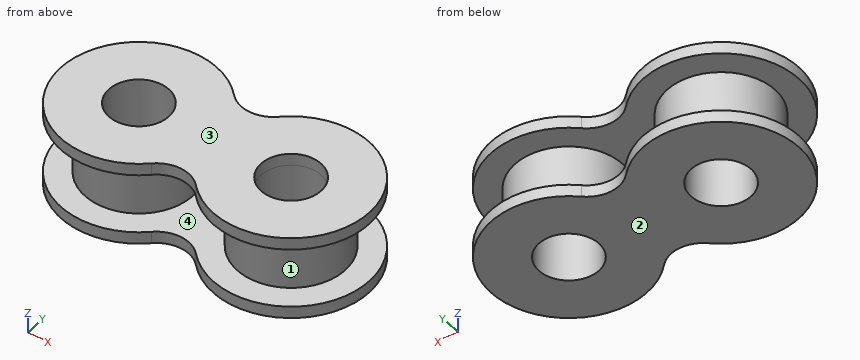
from build123d import *

# Parameters (mm, degrees)
CROQUIS1_R              = 2.5
SALIENTE_EXTRUIR1_DEPTH = 1
CROQUIS2_R              = 4.5
CROQUIS2_R_2            = 2.5
SALIENTE_EXTRUIR2_DEPTH = 5


with BuildPart() as part:
    # Croquis1 → Saliente-Extruir1 (new body)
    with BuildSketch(Plane.XY):
        with BuildLine():
            ThreePointArc((-1.903805922, 4.596194078), (-13, 0), (-1.903805922, -4.596194078))
            ThreePointArc((-1.903805922, -4.596194078), (0, -3.807611845), (1.903805922, -4.596194078))
            ThreePointArc((1.903805922, -4.596194078), (13, 0), (1.903805922, 4.596194078))
            ThreePointArc((1.903805922, 4.596194078), (0, 3.807611845), (-1.903805922, 4.596194078))
        make_face()
        with Locations((-6.5, 0)):
            Circle(CROQUIS1_R, mode=Mode.SUBTRACT)
        with Locations((6.5, 0)):
            Circle(CROQUIS1_R, mode=Mode.SUBTRACT)
    saliente_extruir1 = extrude(amount=SALIENTE_EXTRUIR1_DEPTH)

    # Croquis2 → Saliente-Extruir2 (add)
    with BuildSketch(Plane.XY.offset(1)):
        with Locations((6.5, 0)):
            Circle(CROQUIS2_R)
        with Locations((6.5, 0)):
            Circle(CROQUIS2_R_2, mode=Mode.SUBTRACT)
        with Locations((-6.5, 0)):
            Circle(CROQUIS2_R)
        with Locations((-6.5, 0)):
            Circle(CROQUIS2_R_2, mode=Mode.SUBTRACT)
    extrude(amount=SALIENTE_EXTRUIR2_DEPTH)

    # Simetría1: Saliente-Extruir1 across plane
    add(saliente_extruir1.mirror(Plane.XY.offset(3.5)))


solid = part.part
Can you work these out from the model? Positions are in its coordinate system, mm. Face numbers are marked on the shaded views. A direction names the side the tool comes from. Round coordinates to 2 decimals unless told otherwise and drop trailing zeros. Write each loop counter-clockwise with the first axis right and the second up, starting at its lowest first coordinate (ties: lowest second). Pieces come first, ordered by that corner, then holes. Notation, with made-up numbers: (6, 11.25) -> (19, 11.25) arc R7 cw to (19, 18.25) -> close; hole circle Ø1 at (-11, 45). An arc over 180 degrees is marked (long way). Use one line per item in the form item = value. Start each with the question number.
Q1. Which directions (+Z, -Z, +X, -X, +Y, -Y) give clear straight access to the entire face, cutting with the end or side of a thin tool? Please do the marked faces 3 and 4.
Q2. Imagine slicing it at C-C (z = 6.75). Please give me the cut outline in (x, y), then the cut area to 3 significant figures.
Q3. Imagine slicing it at D-D (y = 3.25). Please give me the cut outline in (x, z), then the cut area to 3 significant figures.
Q4. We'd pull the mould along X, two halves only. Please class the marked faces 1 and 2: +X half, -X half, draft (parallel to the pull), parting line (faces both ways), or undercut.
Q5. Imagine slicing it at B-B (x = 6.5). Please give me the cut outline in (y, z), then the cut area to 3 significant figures.
Q6. Imagine slicing it at A-A (y = -0.75). Please give me the cut outline in (x, z).
Q7. I'm going to push flat-ended pins straight in: P1, Ø2, axis at x = 9.5, z = 6, coming from the +Y side; P2, Ø4, axis at x = 6.5, y = 0, coming from the +Z side. Where does each tip first touch, or does it pass through?
Q8. If I drill on probe 1 along Z at (x, y) = (-2, 4.5); probe 2 along X at (y, z) = (-2, 5); probe 3 along Y at (x, z) = (6.5, 3.8), over which ranges is the centre line in solid material (lowest first)? Write a range as [from, to].
Worked out:
q1.face_3 = +Z, +X, -X, +Y, -Y
q1.face_4 = none
q2.outline = (-1.9, -4.6) arc R2.69 cw to (1.9, -4.6) arc R6.5 ccw (long way) to (1.9, 4.6) arc R2.69 cw to (-1.9, 4.6) arc R6.5 ccw (long way) to start; hole circle Ø5 at (-6.5, 0); hole circle Ø5 at (6.5, 0)
q2.area = 233 mm^2
q3.outline = (-12.13, 0) -> (12.13, 0) -> (12.13, 1) -> (9.61, 1) -> (9.61, 6) -> (12.13, 6) -> (12.13, 7) -> (-12.13, 7) -> (-12.13, 6) -> (-9.61, 6) -> (-9.61, 1) -> (-12.13, 1) -> close; hole (-3.39, 1) -> (3.39, 1) -> (3.39, 6) -> (-3.39, 6) -> close
q3.area = 111 mm^2
q4.face_1 = undercut
q4.face_2 = draft
q5.outline = (-6.5, 0) -> (-2.5, 0) -> (-2.5, 7) -> (-6.5, 7) -> (-6.5, 6) -> (-4.5, 6) -> (-4.5, 1) -> (-6.5, 1) -> close; (2.5, 0) -> (6.5, 0) -> (6.5, 1) -> (4.5, 1) -> (4.5, 6) -> (6.5, 6) -> (6.5, 7) -> (2.5, 7) -> close
q5.area = 36.0 mm^2
q6.outline = (-12.96, 0) -> (-8.88, 0) -> (-8.88, 7) -> (-12.96, 7) -> (-12.96, 6) -> (-10.94, 6) -> (-10.94, 1) -> (-12.96, 1) -> close; (-4.12, 0) -> (4.12, 0) -> (4.12, 7) -> (-4.12, 7) -> close; (8.88, 0) -> (12.96, 0) -> (12.96, 1) -> (10.94, 1) -> (10.94, 6) -> (12.96, 6) -> (12.96, 7) -> (8.88, 7) -> close; hole (-2.06, 1) -> (2.06, 1) -> (2.06, 6) -> (-2.06, 6) -> close
q7.P1 = 6.18
q7.P2 = through
q8.probe_1 = [0, 1], [6, 7]
q8.probe_2 = [-10.53, -8], [-5, -2.47], [2.47, 5], [8, 10.53]
q8.probe_3 = [-4.5, -2.5], [2.5, 4.5]
